CAD build for the part. Positions are in the model's coordinates, mm. A direction names the side the tool comes from. Coordinates: 2 decimals unless noted, no trailing zeros. Write each loop counter-clockwise with the first axis right and the second up, starting at its lowest first coordinate (ties: lowest second). Pieces come first, ordered by that corner, then holes.
```python
from build123d import *

# Parameters (mm, degrees)
SKETCH2_R           = 5
SKETCH2_R_2         = 7.5
SKETCH2_R_3         = 7.07534444
SKETCH2_R_4         = 6.65068888
SKETCH2_R_5         = 6.226033319
SKETCH2_R_6         = 5.801377759
SKETCH2_R_7         = 5.376722199
BOSS_EXTRUDE1_DEPTH = 15
SKETCH3_R           = 0.5
CUT_EXTRUDE2_DEPTH  = 144.75069455
FILLET1_R           = 1
FILLET3_R           = 1
SKETCH4_R           = 2
CUT_EXTRUDE3_DEPTH  = 9


with BuildPart() as part:
    # Sketch2 → Boss-Extrude1 (new body)
    with BuildSketch(Plane(origin=(0, 0, 0), x_dir=(0, 0, -1), z_dir=(1, 0, 0))):
        with BuildLine():
            Line((0, 0), (-6.7, 0))
            Line((-6.7, 0), (-6.7, -3))
            Line((-6.7, -3), (-9.7, -3))
            Line((-9.7, -3), (-9.7, 6))
            Line((-9.7, 6), (35.650511948, 125.510935717))
            ThreePointArc((35.650511948, 125.510935717), (48.253306586, 131.419112363), (54.553243165, 119.007513631))
            Line((54.553243165, 119.007513631), (10, -25))
            Line((10, -25), (0, -25))
            Line((0, -25), (0, 0))
        make_face()
        with Locations((45, 121.963109177)):
            Circle(SKETCH2_R, mode=Mode.SUBTRACT)
        with Locations((10.525284468, 21.759512837)):
            Circle(SKETCH2_R_2, mode=Mode.SUBTRACT)
        with Locations((16.381236323, 38.780318572)):
            Circle(SKETCH2_R_3, mode=Mode.SUBTRACT)
        with Locations((22.237188178, 55.801124308)):
            Circle(SKETCH2_R_4, mode=Mode.SUBTRACT)
        with Locations((28.093140033, 72.821930043)):
            Circle(SKETCH2_R_5, mode=Mode.SUBTRACT)
        with Locations((33.949091887, 89.842735778)):
            Circle(SKETCH2_R_6, mode=Mode.SUBTRACT)
        with Locations((39.805043742, 106.863541513)):
            Circle(SKETCH2_R_7, mode=Mode.SUBTRACT)
    extrude(amount=BOSS_EXTRUDE1_DEPTH)

    # Sketch3 → Cut-Extrude2 (cut, through all)
    with BuildSketch(Plane(origin=(0, 0, 0), x_dir=(0, 0, -1), z_dir=(1, 0, 0))):
        Circle(SKETCH3_R)
        with Locations((-6.7, 0)):
            Circle(SKETCH3_R)
    extrude(amount=CUT_EXTRUDE2_DEPTH, mode=Mode.SUBTRACT)

    # Fillet1
    fillet1_edges = [part.edges().sort_by_distance(p)[0] for p in [
        (7.5, -3, 6.7),
        (7.5, -3, 9.7),
        (7.5, -0.5, 0),
        (7.5, 0, 6.2),
        (7.5, 0, 0.5),
        (7.5, -0.5, 6.7),
    ]]
    fillet(fillet1_edges, radius=FILLET1_R)

    # Fillet3
    fillet3_edges = [part.edges().sort_by_distance(p)[0] for p in [
        (7.5, -25, -10),
        (7.5, -25, 0),
    ]]
    fillet(fillet3_edges, radius=FILLET3_R)

    # Sketch4 → Cut-Extrude3 (cut)
    with BuildSketch(Plane.XZ.offset(25)):
        with Locations(Location((7.5, -5, 0), (0, 0, 270))):
            Circle(SKETCH4_R)
    extrude(amount=-CUT_EXTRUDE3_DEPTH, mode=Mode.SUBTRACT)


solid = part.part
```
Item 1: Two-plate mould, pull along Z, no slides. Class faces 4 (the flat face through (7.4, 64.92, -12.66)), 5 (the cylindrical face through (7.395, 31.873, -14.847)), 6 (the cylindrical face through (7.395, 131.487, -48.049)): +Z half, -Z half, draft (parallel to the pull), parting line (faces both ways), or undercut.
Item 2: Saw through at C-C, the plane x = 1.5. Write the cut outline in (y, z), and give its area (3 significant figures).
Item 3: Wall check: line 1 along Z through (x, y) = (2.25, 54); line 2 along Z through (x, y) = (3.5, 39); line 3 along Z through (x, y) = (4, 66.5). Give the ranges that are in metal, low to high.
Item 4: Saw through at B-B, the plane y = 19. Write the cut outline in (x, z).
Item 5: Saw through at A-A, the plane z = -5. Write the cut outline in (x, y), and give its area (3 significant figures).
Item 6: Which spindle directions (+Z, -Z, +X, -X, +Y, -Y) get a long thin tool onto all of the face, cutting with end or side? Do faces 1 (the cylindrical face through (7.4, 126.92, -44.35)), 2 (the flat face through (7, 0, 3)), 3 (the cylindrical face through (8.852, -20.563, -3.526)). Say none if no direction does.
Item 7: Saw through at D-D, the plane z = -20. Write the cut outline in (x, y), and give its area (3 significant figures).
Item 8: Flat gauge pins, fed straight in: pin 1 Ø6 at (x, z) = (1.5, -13) entering from -Y; pin 2 Ø9.5 at (y, z) = (106.86, -39.81) entering from -X; pin 3 Ø7.5 at (x, y) = (8, -17.5) entering from +Z; pin 4 Ø5 at (x, z) = (6, 3.5) entering from -Y. Where does each tip first touch, or does it go through?
Working result:
1. face 4: +Z half
1. face 5: undercut
1. face 6: parting line
2. outline: (-25, -9.26) arc R1 ccw to (-24.3, -10.22) - (119.01, -54.55) arc R10 ccw to (125.51, -35.65) - (6, 9.7) - (-2, 9.7) arc R1 ccw to (-3, 8.7) - (-3, 7.7) arc R1 ccw to (-2, 6.7) - (-1.12, 6.7) arc R1 ccw to (-0.37, 7.03) arc R0.5 cw (long way) to (0.33, 6.33) arc R1 ccw to (0, 5.58) - (0, 1.12) arc R1 ccw to (0.33, 0.37) arc R0.5 cw (long way) to (-0.37, -0.33) arc R1 ccw to (-1.12, 0) - (-24, 0) arc R1 ccw to (-25, -1) - close; hole circle Ø15 at (21.76, -10.53); hole circle Ø14.15 at (38.78, -16.38); hole circle Ø13.3 at (55.8, -22.24); hole circle Ø12.45 at (72.82, -28.09); hole circle Ø11.6 at (89.84, -33.95); hole circle Ø10.75 at (106.86, -39.81); hole circle Ø10 at (121.96, -45)
2. area: 2,740 mm2
3. line 1: z = -34.44 to -28.64, -15.84 to -8.51
3. line 2: z = -29.8 to -23.45, -9.31 to -2.82
3. line 3: z = -38.31 to -13.26
4. outline: (0, -23.61) - (15, -23.61) - (15, -17.5) - (0, -17.5) - close; (0, -3.55) - (15, -3.55) - (15, 4.77) - (0, 4.77) - close
5. outline: (0, -25) - (5.5, -25) - (5.5, -16) - (9.5, -16) - (9.5, -25) - (15, -25) - (15, 16.69) - (0, 16.69) - close; (0, 26.83) - (15, 26.83) - (15, 44.74) - (0, 44.74) - close
5. area: 858 mm2
6. face 1: +X, -X
6. face 2: +X, -X, -Y
6. face 3: -Y
7. outline: (0, 7.32) - (15, 7.32) - (15, 32.7) - (0, 32.7) - close; (0, 44.86) - (15, 44.86) - (15, 49.54) - (0, 49.54) - close; (0, 62.06) - (15, 62.06) - (15, 84.27) - (0, 84.27) - close
7. area: 784 mm2
8. pin 1: stops at y = -24.68
8. pin 2: passes through
8. pin 3: stops at z = 0
8. pin 4: stops at y = 0
